Autodesk Inventor part; units mm, degrees
ref_plane "YZ Plane" through (0, 0, 0) normal (1, 0, 0) x (0, 1, 0)
ref_plane "XZ Plane" through (0, 0, 0) normal (0, 1, 0) x (-1, 0, 0)
ref_plane "XY Plane" through (0, 0, 0) normal (0, 0, 1) x (1, 0, 0)
sketch "Sketch1" plane through (0, 0, 0) normal (0, 0, 1) x (1, 0, 0)
  circle A0 centre (0, 0) radius 6.35 construction
  circle A1 centre (-52.07, 0) radius 45.72 construction
  circle A2 centre (-52.07, 0) radius 12.7 construction
  circle A3 centre (-52.07, 54.61) radius 41.91 construction
  circle A4 centre (-52.07, 54.61) radius 12.7 construction
  circle A5 centre (2.54, 54.61) radius 41.91 construction
  line L0 (-97.79, 96.52) -> (44.45, 96.52)
  line L1 (44.45, 96.52) -> (44.45, -45.72)
  line L2 (44.45, -45.72) -> (-97.79, -45.72)
  line L3 (-97.79, -45.72) -> (-97.79, 96.52)
  circle A6 centre (0, 0) radius 25.4 construction
  point P0 (25.4, 0)
  point P1 (21.997, 12.7)
  point P2 (12.7, 21.997)
  point P3 (0, 25.4)
  point P4 (-12.7, 21.997)
  point P5 (-21.997, 12.7)
  point P6 (-25.4, 0)
  point P7 (-21.997, -12.7)
  point P8 (-12.7, -21.997)
  point P9 (0, -25.4)
  point P10 (12.7, -21.997)
  point P11 (21.997, -12.7)
  dimension "d15" = 50.8
  dimension "d0" = 12.7
  dimension "d1" = 91.44
  dimension "d2" = 25.4
  dimension "d3" = 83.82
  dimension "d4" = 25.4
  dimension "d5" = 83.82
  dimension "d18" = 360
extrude "Extrusion1" add sketch "Sketch1" against normal blind 6.35
hole "Hole1" at (-52.07, 0, 0) at (2.54, 54.61, 0) at (-52.07, 54.61, 0) direction (0, 0, -1) diameter 28.575 end through all
hole "Hole2" at (25.4, 0, 0) at (21.997, 12.7, 0) at (12.7, 21.997, 0) at (0, 25.4, 0) at (-12.7, 21.997, 0) at (-21.997, 12.7, 0) at (-25.4, 0, 0) at (-21.997, -12.7, 0) at (-12.7, -21.997, 0) at (0, -25.4, 0) at (12.7, -21.997, 0) at (21.997, -12.7, 0) direction (0, 0, -1) diameter 5.1054 end through all
hole "Hole3" at (0, 0, 0) direction (0, 0, -1) diameter 20.955 end through all
properties part number "CL4-014" material "Aluminum 6061"
Input: part model. Units: mm. Frame: model coordinates. Coordinates: 2 decimals unless noted, no trailing zeros. Order: outer loops, then holes, each group sorted by start corner. A loop starts at its lowest first (then second) coordinate and runs counter-clockwise, first axis right, second up. Notation, with made-up numbers: (-3.75, 55) - (9.25, 55) arc R32 ccw to (9.25, 83) - close; hole circle Ø9 at (20, 12). An arc over 180 degrees is marked (long way). Put each result on its own line as item: value.
1. Line query: line 1 along X through (y, z) = (54.61, -2.5); line 2 along X through (y, z) = (0, -3.25); line 3 along X through (y, z) = (2, -3). Output: solid intervals per line, ascending.
Report:
line 1: x = -97.79 to -66.36, -37.78 to -11.75, 16.83 to 44.45
line 2: x = -97.79 to -66.36, -37.78 to -27.95, -22.85 to -10.48, 10.48 to 22.85, 27.95 to 44.45
line 3: x = -97.79 to -66.22, -37.92 to -26.99, -23.81 to -10.28, 10.28 to 23.81, 26.99 to 44.45
2. Cut plane C-C on z = -1.5. State how many separate pieces and enclosed holes the cut face has, then the cut area to 3 significant figures.
Report:
separate pieces: 1
enclosed holes: 16
area: 17,700 mm2
3. Draft query along X for faces 1 (the face through (-97.79, 24, -3)), 2 (the face through (19.845, 11.328, -3.219)), 3 (the face through (-28, 26, 0)). Return one class per face: pulls with the +X half, pulls with the -X half, needs draft (parallel to the pull), parting line crosses it, or undercut.
Report:
face 1: pulls with the -X half
face 2: undercut
face 3: needs draft
4. Cut plane D-D on x = -56.5. Return the cut outline in (y, z).
Report:
outline: (-45.72, -6.35) - (-13.58, -6.35) - (-13.58, 0) - (-45.72, 0) - close; (13.58, -6.35) - (41.03, -6.35) - (41.03, 0) - (13.58, 0) - close; (68.19, -6.35) - (96.52, -6.35) - (96.52, 0) - (68.19, 0) - close
5. Contact query for a flat-ended pin moving along its axis: pin 1 Ø3 at (x, y) = (-12.7, 21.997) entering from +Z. Output: stop coordinate, or through.
Report:
pin 1: passes through
6. Cut plane A-A on x = 0. Return the cut outline in (y, z), then the cut area to 3 significant figures.
Report:
outline: (-45.72, -6.35) - (-27.95, -6.35) - (-27.95, 0) - (-45.72, 0) - close; (-22.85, -6.35) - (-10.48, -6.35) - (-10.48, 0) - (-22.85, 0) - close; (10.48, -6.35) - (22.85, -6.35) - (22.85, 0) - (10.48, 0) - close; (27.95, -6.35) - (40.55, -6.35) - (40.55, 0) - (27.95, 0) - close; (68.67, -6.35) - (96.52, -6.35) - (96.52, 0) - (68.67, 0) - close
area: 527 mm2
7. Cut plane B-B on y = 44.5. Return the cut outline in (x, z), then the cut area to 3 significant figures.
Report:
outline: (-97.79, -6.35) - (-62.17, -6.35) - (-62.17, 0) - (-97.79, 0) - close; (-41.97, -6.35) - (-7.56, -6.35) - (-7.56, 0) - (-41.97, 0) - close; (12.64, -6.35) - (44.45, -6.35) - (44.45, 0) - (12.64, 0) - close
area: 647 mm2
